Autodesk Inventor part; units mm, degrees
ref_plane "YZ Plane" through (0, 0, 0) normal (1, 0, 0) x (0, 1, 0)
ref_plane "XZ Plane" through (0, 0, 0) normal (0, 1, 0) x (-1, 0, 0)
ref_plane "XY Plane" through (0, 0, 0) normal (0, 0, 1) x (1, 0, 0)
sketch "スケッチ1" plane through (0, 0, 0) normal (0, 1, 0) x (-1, 0, 0)
  line L0 (-7.5, -7.5) -> (7.5, -7.5)
  line L1 (7.5, -7.5) -> (7.5, 7.5)
  line L2 (7.5, 7.5) -> (-7.5, 7.5)
  line L3 (-7.5, 7.5) -> (-7.5, -7.5)
  line L4 (-7.5, -7.5) -> (7.5, 7.5) construction
  line L5 (7.5, -7.5) -> (-7.5, 7.5) construction
  point P0 (0, 0)
  dimension "d0" = 15
extrude "押し出し1" add sketch "スケッチ1" along normal blind 460
shell "シェル1" thickness 1 removed faces 2 at (2.5, 0, 2.5) at (2.5, 460, 2.5)
sketch "スケッチ2" plane through (7.5, 0, -7.5) normal (0, 0, -1) x (-1, 0, 0)
  line L0 (7.5, 0) -> (7.5, 70) construction
  line L1 (0, 460) -> (15, 460)
  point P0 (7.5, 107)
  point P1 (7.5, 452.5)
  dimension "d4" = 37
  dimension "d5" = 70
  dimension "d13" = 7.5
hole "穴1" at (0, 70, -7.5) at (0, 107, -7.5) at (0, 452.5, -7.5) direction (0, 0, 1) diameter 3.2 end through all
properties part number "BaseSupportSQpipe"
Could you check a few things on this model? Use its own coordinates, in mm. A direction names the side the tool comes from. Give positions to 0.01 mm unless a question says otherwise; leave off trailing zeros. Order: outer loops, then holes, each group sorted by start corner. A loop starts at its lowest first (then second) coordinate and runs counter-clockwise, first axis right, second up. Notation, with made-up numbers: (4.5, -25.5) - (33.5, -25.5) arc R16 ccw to (33.5, 4.5) - close; hole circle Ø10 at (-30.75, 17.25). An arc over 180 degrees is marked (long way). One line per question, with ' | ' between items. Start each with the question number.
Item 1: I want a section at B-B on z = 0.25. Write out the boundary of the cut face in (x, y), then the cut area to 3 significant figures.
Item 2: Thinking about a two-plate mould opening in X: for faces 3 (the flat face through (0, 227, 7.5)), 4 (the flat face through (-6.5, 227, 0)), 5 (the flat face through (7.5, 227, 0)), which applies, pulls with the +X half, pulls with the -X half, needs draft (parallel to the pull), parting line crosses it, or undercut?
Item 3: For faces 1 (the flat face through (-7.5, 227, 0)), 2 (the flat face through (6.5, 227, 0)), which set-ups out of +Z, -Z, +X, -X, +Y, -Y let a thin tool reach every point of the face, with its end or its side?
Item 4: I'm going to push a flat-ended pin straight in: pin 1 Ø1.9 at (x, y) = (0, 107) entering from -Z. Where does the tip first touch, or does it pass through?
Item 5: I need wall thicknesses on probe 1 along Z at (x, y) = (3.5, 177.5); probe 2 along X at (y, z) = (107, -6.75). Which ranges of each line are inside material? Lowest first, please. Write a range as [from, to].
Item 6: I want a section at A-A on x = 4. Write out the boundary of the cut face in (y, z), then the cut area to 3 significant figures.
Item 7: I want a section at C-C on y = 80.5. Write out the boundary of the cut face in (x, z), then the cut area to 3 significant figures.
Verdict:
1) outline: (-7.5, 0) - (-6.5, 0) - (-6.5, 460) - (-7.5, 460) - close; (6.5, 0) - (7.5, 0) - (7.5, 460) - (6.5, 460) - close | area: 920 mm^2
2) face 3: needs draft | face 4: undercut | face 5: pulls with the +X half
3) face 1: +Z, -Z, -X, +Y, -Y | face 2: +Y, -Y
4) pin 1: through
5) probe 1: [-7.5, -6.5], [6.5, 7.5] | probe 2: [-7.5, -1.6], [1.6, 7.5]
6) outline: (0, -7.5) - (460, -7.5) - (460, -6.5) - (0, -6.5) - close; (0, 6.5) - (460, 6.5) - (460, 7.5) - (0, 7.5) - close | area: 920 mm^2
7) outline: (-7.5, -7.5) - (7.5, -7.5) - (7.5, 7.5) - (-7.5, 7.5) - close; hole (-6.5, -6.5) - (6.5, -6.5) - (6.5, 6.5) - (-6.5, 6.5) - close | area: 56.0 mm^2
